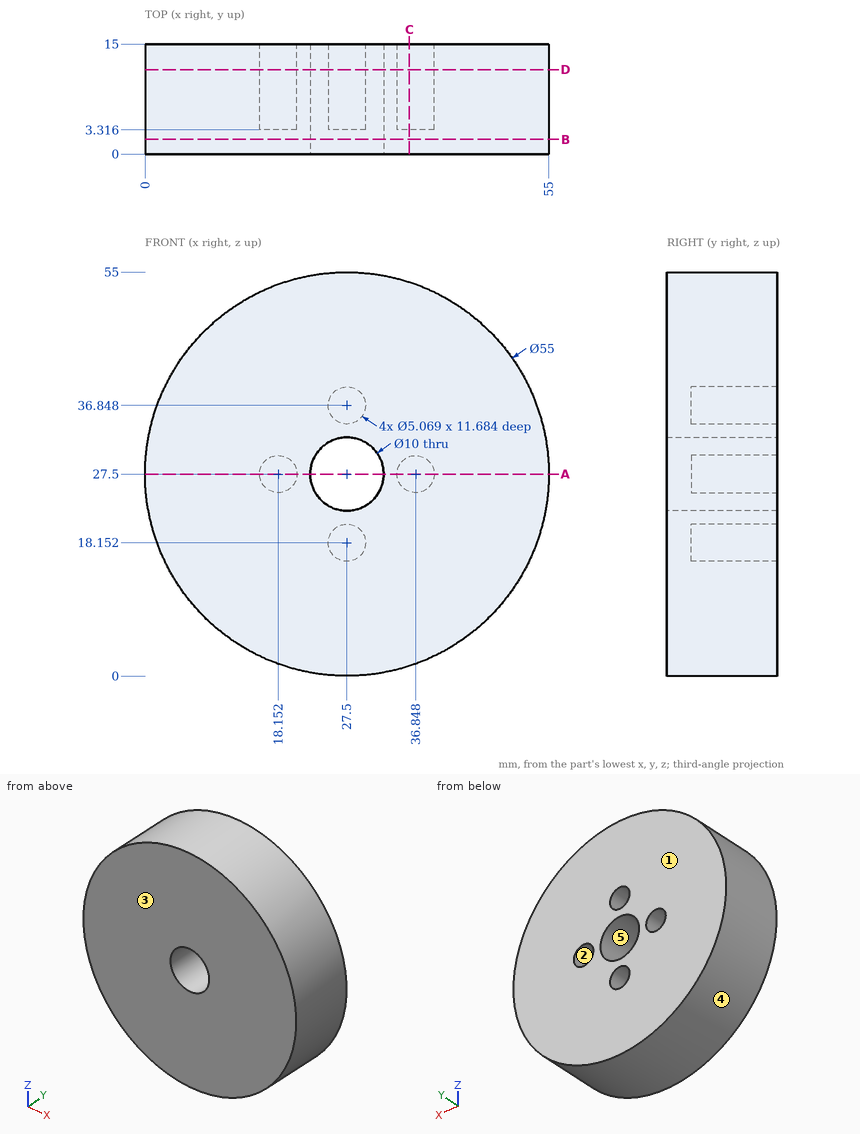
Print and shaded views of the part. All mm, measured from the part's lowest x, y and z. A direction names the side the tool comes from. Coordinates: 2 decimals unless noted, no trailing zeros. Loops run counter-clockwise (first coordinate to the right, second up) from the corner with the lowest first, then second, coordinate; pieces in that order, holes last. Notation, with made-up numbers: (68, 11) -> (115, 11) arc R11 ccw to (115, 20) -> close; hole circle Ø2 at (-33.5, 45). An arc over 180 degrees is marked (long way). Use one line per item in the form item = value. Start each with the question number.
(1) Cut at B-B on y = 2. Give the cut face in (x, z), and give its area (3 significant figures).
(2) Tool access for the marked faces 1 and 2: list every direction of +Z, -Z, +X, -X, +Y, -Y with a clear straight run to the whole face (end or side of a thin tool).
(3) Cut at C-C on x = 36. Give the cut face in (y, z).
(4) Pull direction Z, two halves, no side cores. Call the marked faces 3, 4 and 5: pulls with the +Z half, pulls with the -Z half, needs draft (parallel to the pull), parting line crosses it, or undercut.
(5) Cut at A-A on z = 27.5. Give the cut face in (x, y).
(6) Probe probe 1 along X at (y, z) = (9.5, 27.5); probe 2 along X at (y, z) = (14, 24.5) (1 decimal). List the from-to ranges inside material, lowest first. Write a range as from..to.
(7) Flat gauge pins, fed straight in: pin 1 (2 mm diameter, centred on y = 8.5, z = 10, fed in from -X); pin 2 (1.5 mm diameter, centred on x = 18, z = 27, fed in from +Y); pin 3 (6 mm diameter, centred on x = 19, y = 9, fed in from -Z). Where does each tip first touch, or does it go through?
(8) Cut at D-D on y = 11.5. Give the cut face in (x, z) (1 decimal).
Values:
q1.outline = circle Ø55 at (27.5, 27.5); hole circle Ø10 at (27.5, 27.5)
q1.area = 2,300 mm2
q2.face_1 = +Z, -Z, +X, -X, +Y
q2.face_2 = +Y
q3.outline = (0, 1.35) -> (15, 1.35) -> (15, 25.11) -> (3.32, 25.11) -> (3.32, 29.89) -> (15, 29.89) -> (15, 53.65) -> (0, 53.65) -> close
q4.face_3 = needs draft
q4.face_4 = parting line crosses it
q4.face_5 = undercut
q5.outline = (0, 0) -> (22.5, 0) -> (22.5, 15) -> (20.69, 15) -> (20.69, 3.32) -> (15.62, 3.32) -> (15.62, 15) -> (0, 15) -> close; (32.5, 0) -> (55, 0) -> (55, 15) -> (39.38, 15) -> (39.38, 3.32) -> (34.31, 3.32) -> (34.31, 15) -> (32.5, 15) -> close
q6.probe_1 = 0..15.62, 20.69..22.5, 32.5..34.31, 39.38..55
q6.probe_2 = 0.2..23.5, 31.5..54.8
q7.pin_1 = 5.5
q7.pin_2 = 3.32
q7.pin_3 = 0.56
q8.outline = circle Ø55 at (27.5, 27.5); hole circle Ø5.1 at (18.2, 27.5); hole circle Ø10 at (27.5, 27.5); hole circle Ø5.1 at (27.5, 18.2); hole circle Ø5.1 at (27.5, 36.8); hole circle Ø5.1 at (36.8, 27.5)
